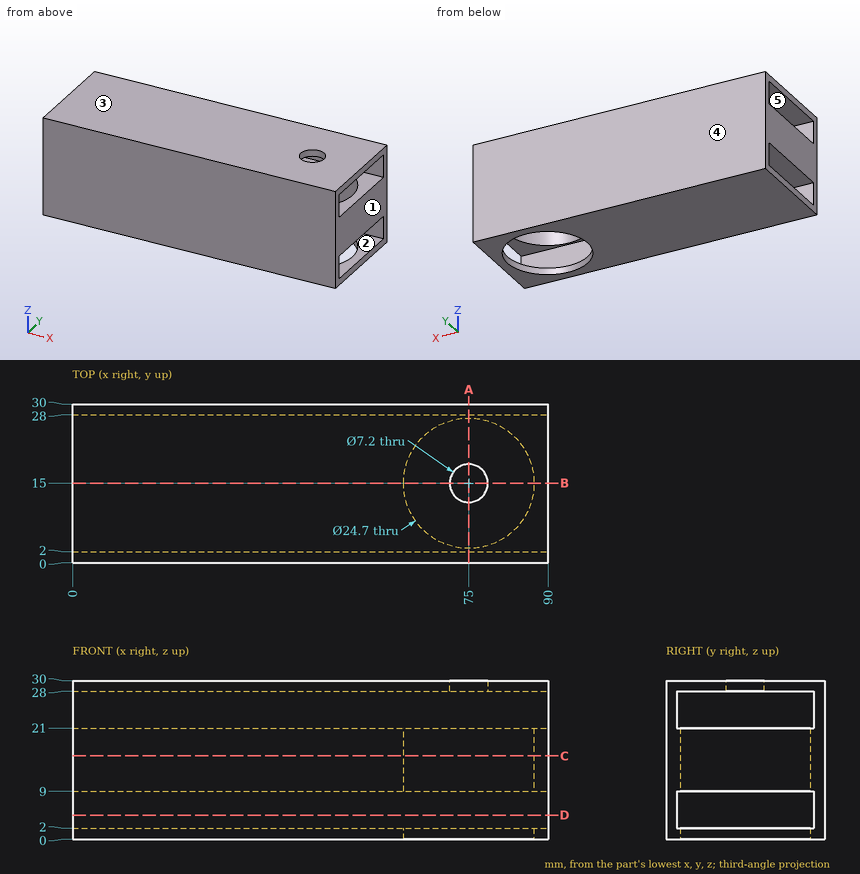
Print and shaded views of the part. All mm, measured from the part's lowest x, y and z. A direction names the side the tool comes from. Coordinates: 2 decimals unless noted, no trailing zeros. Order: outer loops, then holes, each group sorted by start corner. A loop starts at its lowest first (then second) coordinate and runs counter-clockwise, first axis right, second up. Notation, with made-up numbers: (75.25, 27.25) - (117.25, 27.25) arc R21 cw to (117.25, 56.25) - close; hole circle Ø3 at (70.5, -8). An arc over 180 degrees is marked (long way). Return JSON: item names as keys, results as strings. Group by question number.
Item 1: Cut at B-B (y = 15). List the corners of the cut face in (x, z).
Item 2: Which spindle directions (+Z, -Z, +X, -X, +Y, -Y) get a long thin tool onto all of the face, cutting with end or side? Do the marked faces 4 and 5. Say none if no direction does.
Item 3: Cut at A-A (x = 75). List the corners of the cut face in (y, z), plus the area to 3 significant figures.
Item 4: Cut at C-C (z = 15.75). List the corners of the cut face in (x, y), plus the area to 3 significant figures.
Item 5: Drill centre lines: probe 1 along Z at (x, y) = (7.5, 20.25); probe 2 along Y at (x, z) = (21.5, 3.5); probe 3 along Y at (x, z) = (75, 0.85). Where is each one in solid material? Low to high. Write a range as from..to.
Item 6: Pull direction Z, two halves, no side cores. Call the marked faces 1, 2 and 3: pulls with the +Z half, pulls with the -Z half, needs draft (parallel to the pull), parting line crosses it, or undercut.
Item 7: Cut at D-D (z = 4.5). List the corners of the cut face in (x, y).
Item 8: Pin check, flat tip, straight feed: pin 1 (4 mm diameter, centred on x = 79.5, y = 15.5, fed in from -Z). Stop position of the tip, or through.
Check values:
{
 "1": {"outline": "(0, 0) - (62.65, 0) - (62.65, 2) - (0, 2) - close; (0, 9) - (62.65, 9) - (62.65, 21) - (0, 21) - close; (0, 28) - (71.4, 28) - (71.4, 30) - (0, 30) - close; (78.6, 28) - (90, 28) - (90, 30) - (78.6, 30) - close; (87.35, 0) - (90, 0) - (90, 2) - (87.35, 2) - close; (87.35, 9) - (90, 9) - (90, 21) - (87.35, 21) - close"},
 "2": {"face 4": "+Z, -Z, +X, -X, +Y", "face 5": "+X, -X"},
 "3": {"outline": "(0, 0) - (2.65, 0) - (2.65, 2) - (2, 2) - (2, 9) - (2.65, 9) - (2.65, 21) - (2, 21) - (2, 28) - (11.4, 28) - (11.4, 30) - (0, 30) - close; (18.6, 28) - (28, 28) - (28, 21) - (27.35, 21) - (27.35, 9) - (28, 9) - (28, 2) - (27.35, 2) - (27.35, 0) - (30, 0) - (30, 30) - (18.6, 30) - close", "area": "176 mm2"},
 "4": {"outline": "(0, 0) - (90, 0) - (90, 30) - (0, 30) - close; hole circle Ø24.7 at (75, 15)", "area": "2,220 mm2"},
 "5": {"probe 1": "z = 0..2, 9..21, 28..30", "probe 2": "y = 0..2, 28..30", "probe 3": "y = 0..2.65, 27.35..30"},
 "6": {"face 1": "needs draft", "face 2": "undercut", "face 3": "pulls with the +Z half"},
 "7": {"outline": "(0, 0) - (90, 0) - (90, 2) - (0, 2) - close; (0, 28) - (90, 28) - (90, 30) - (0, 30) - close"},
 "8": {"pin 1": "stops at z = 28"}
}
